The listing builds one solid part. Answer for the finished solid, in the listing's coordinates (mm). A direction names the side the tool comes from. Give positions to 0.01 mm unless a question says otherwise; leave off trailing zeros. Order: outer loops, then holes, each group sorted by start corner. A loop starts at its lowest first (then second) coordinate and runs counter-clockwise, first axis right, second up. Notation, with made-up numbers: (15.25, 25.5) - (44.25, 25.5) arc R14 cw to (44.25, 48.5) - close; hole circle Ø9 at (62, -31.75). An arc over 180 degrees is marked (long way). Use a Markdown table: item, result. Add a question column.
1) For faces 4 (the face through (38, 17.526, -13)), 5 (the face through (38, 7.874, -13)), 6 (the face through (37.567, 7.614, -5.137)), 7 (the face through (38, 16.002, -24)), determine the directions among +Z, -Z, +X, -X, +Y, -Y from which every point of the face is accessible in a straight line to the end or side of a thin tool.
2) The mould has two halves that part along Y. Classify faces 1 (the face through (38, 22.924, -18)), 2 (the face through (38, 0, -21)), 3 (the face through (38, 5, 0)): released by +Y, released by -Y, zero draft, split by the parting line, or undercut.
3) Find section B-B, the plane z = -12.7. Determine the outline of the cut face in (x, y), plus the area to 3 significant figures.
4) Find section C-C, the plane y = 16.75. Determine the outline of the cut face in (x, z), plus the area to 3 significant figures.
5) Flat-ended cylindrical pins translate along their axes: pin 1 (4 mm diameter, centred on x = 53, y = 13.5, fed in from -Z); pin 2 (1.4 mm diameter, centred on x = 56.5, y = 13.5, fed in from +Z); pin 3 (5 mm diameter, centred on y = 11.5, z = -21.5, fed in from -X). Find the tip coordinate at first contact, or state that the pin passes through.
6) Find section A-A, the plane y = 12.7. Determine the outline of the cut face in (x, z), plus the area to 3 significant figures.
7) Straight lines are drawn through the part: line 1 (Z direction, x = 40, y = 2); line 2 (Y direction, x = 7, z = -20); line 3 (Z direction, x = 64, y = 6.5). For each, find the intervals that lie inside material, in ascending order.
Autodesk Inventor part; units mm, degrees
ref_plane "YZ Plane" through (0, 0, 0) normal (1, 0, 0) x (0, 1, 0)
ref_plane "XZ Plane" through (0, 0, 0) normal (0, 1, 0) x (-1, 0, 0)
ref_plane "XY Plane" through (0, 0, 0) normal (0, 0, 1) x (1, 0, 0)
sketch "Sketch1" plane through (0, 0, 0) normal (1, 0, 0) x (0, 1, 0)
  line L0 (0, 0) -> (0, -9.398)
  line L1 (0, -9.398) -> (2.4765, -9.398)
  line L2 (9.398, -2.4765) -> (9.398, 0)
  line L3 (9.398, 0) -> (0, 0)
  line L4 (16.002, 0) -> (16.002, -2.4765)
  line L5 (22.9235, -9.398) -> (25.4, -9.398)
  line L6 (25.4, -9.398) -> (25.4, 0)
  line L7 (25.4, 0) -> (16.002, 0)
  line L8 (25.4, -16.002) -> (22.9235, -16.002)
  line L9 (16.002, -22.9235) -> (16.002, -25.4)
  line L10 (16.002, -25.4) -> (25.4, -25.4)
  line L11 (25.4, -25.4) -> (25.4, -16.002)
  line L12 (0, -16.002) -> (2.4765, -16.002)
  line L13 (9.398, -22.9235) -> (9.398, -25.4)
  line L14 (9.398, -25.4) -> (0, -25.4)
  line L15 (0, -25.4) -> (0, -16.002)
  line L16 (22.9235, -9.398) -> (22.9235, -4.953)
  line L17 (16.002, -2.4765) -> (20.447, -2.4765)
  line L18 (20.447, -2.4765) -> (15.0495, -7.874)
  line L19 (20.447, -2.4765) -> (28.0802, -2.4765) construction
  line L20 (22.9235, -4.953) -> (17.526, -10.3505)
  line L21 (22.9235, -16.002) -> (22.9235, -20.447)
  line L22 (22.9235, -20.447) -> (17.526, -15.0495)
  line L23 (16.002, -22.9235) -> (20.447, -22.9235)
  line L24 (20.447, -22.9235) -> (15.0495, -17.526)
  line L25 (2.4765, -16.002) -> (2.4765, -20.447)
  line L26 (2.4765, -20.447) -> (7.874, -15.0495)
  line L27 (9.398, -22.9235) -> (4.953, -22.9235)
  line L28 (4.953, -22.9235) -> (10.3505, -17.526)
  line L29 (9.398, -2.4765) -> (4.953, -2.4765)
  line L30 (4.953, -2.4765) -> (10.3505, -7.874)
  line L31 (2.4765, -9.398) -> (2.4765, -4.953)
  line L32 (2.4765, -4.953) -> (7.874, -10.3505)
  line L33 (10.3505, -7.874) -> (15.0495, -7.874)
  line L34 (17.526, -10.3505) -> (17.526, -15.0495)
  line L35 (10.3505, -17.526) -> (15.0495, -17.526)
  line L36 (7.874, -15.0495) -> (7.874, -10.3505)
  circle A0 centre (12.7, -12.7) radius 2.54
  dimension "d2" = 9.398
  dimension "d3" = 2.4765
  dimension "d7" = 2.4765
  dimension "d10" = 2.4765
  dimension "d11" = 25.4
  dimension "d13" = 2.4765
  dimension "d16" = 2.4765
  dimension "d17" = 9.398
  dimension "d18" = 25.4
  dimension "d23" = 2.4765
  dimension "d24" = 25.4
  dimension "d25" = 25.4
  dimension "d32" = 4.445
  dimension "d33" = 4.445
  dimension "d35" = 135
  dimension "d36" = 4.445
  dimension "d37" = 4.445
  dimension "d38" = 2.4765
  dimension "d40" = 4.445
  dimension "d41" = 4.445
  dimension "d42" = 4.445
  dimension "d43" = 4.445
  dimension "d44" = 5.08
extrude "Extrusion1" add sketch "Sketch1" along normal blind 76.2
properties part number "LatX24in1"
The answers:
| question | item | result |
|---|---|---|
| 1 | face 4 | +X, -X, +Y |
| 1 | face 5 | +X, -X, -Y |
| 1 | face 6 | +X, -X |
| 1 | face 7 | -Z, +X, -X |
| 2 | face 1 | undercut |
| 2 | face 2 | released by -Y |
| 2 | face 3 | zero draft |
| 3 | outline | (0, 7.87) - (76.2, 7.87) - (76.2, 10.16) - (0, 10.16) - close; (0, 15.24) - (76.2, 15.24) - (76.2, 17.53) - (0, 17.53) - close |
| 3 | area | 348 mm2 |
| 4 | outline | (0, -25.4) - (76.2, -25.4) - (76.2, -22.92) - (0, -22.92) - close; (0, -19.23) - (76.2, -19.23) - (76.2, -6.17) - (0, -6.17) - close; (0, -2.48) - (76.2, -2.48) - (76.2, 0) - (0, 0) - close |
| 4 | area | 1,370 mm2 |
| 5 | pin 1 | z = -17.98 |
| 5 | pin 2 | z = -7.87 |
| 5 | pin 3 | through |
| 6 | outline | (0, -17.53) - (76.2, -17.53) - (76.2, -15.24) - (0, -15.24) - close; (0, -10.16) - (76.2, -10.16) - (76.2, -7.87) - (0, -7.87) - close |
| 6 | area | 348 mm2 |
| 7 | line 1 | -25.4 to -16, -9.4 to 0 |
| 7 | line 2 | 0 to 2.48, 2.92 to 7.88, 17.52 to 22.48, 22.92 to 25.4 |
| 7 | line 3 | -25.4 to -22.92, -21.38 to -16.42, -8.98 to -4.02, -2.48 to 0 |
